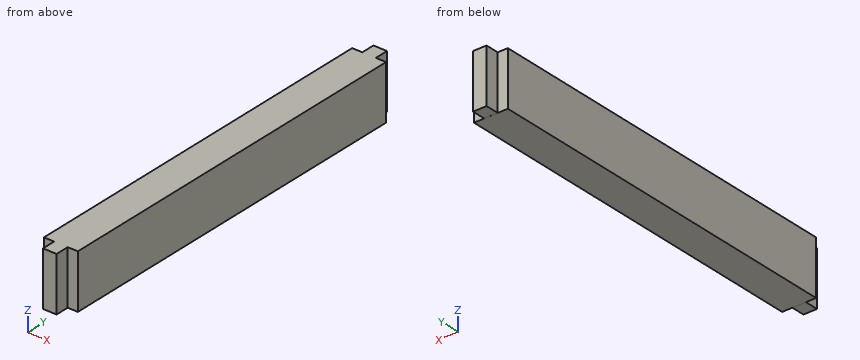
```python
from build123d import *

# Parameters (mm, degrees)
F0_W     = 12.7
F0_H     = 50.77157
F1_DEPTH = 12.7
F2_DEPTH = 365.125
F3_DEPTH = 352.425


with BuildPart() as f1:
    # F0 (on Front) → F1 (new body)
    with BuildSketch(Plane.XZ):
        with Locations((-9.980159, 8.597515)):
            Rectangle(F0_W, F0_H)
    extrude(amount=F1_DEPTH)

    # F0 (on Front) → F2 (join)
    with BuildSketch(Plane.XZ):
        with Locations((-9.980159, 8.597515)):
            Rectangle(F0_W, F0_H)
    extrude(amount=-F2_DEPTH)

    # F0 (on Front) → F3 (join)
    with BuildSketch(Plane.XZ):
        Polygon((-16.330159, 33.9833), (-25.855159, 33.9833), (-25.855159, -16.8167), (5.894841, -16.8167), (5.894841, 33.9833), (-3.630159, 33.9833), (-3.630159, -16.78827), (-16.330159, -16.78827), align=None)
    extrude(amount=-F3_DEPTH)


solid = f1.part
```
CAD build for the part. Positions are in the model's coordinates, mm. Round coordinates to 2 decimals unless told otherwise and drop trailing zeros. Loops run counter-clockwise (first coordinate to the right, second up) from the corner with the lowest first, then second, coordinate; pieces in that order, holes last. Notation, with made-up numbers: M -19,73.5 L -11,73.5 A26 cw -11,105.5 Z; hole C 20.25,-7 d6. An arc over 180 degrees is marked long. Return JSON: item names as keys, results as strings. Group by question number.
(1) Saw through at B-B, the plane x = 2.5. List the corners of the cut face in (y, z) (3 decimals).
(2) Saw through at A-A, the plane z = 6.5. List the corners of the cut face in (x, y) (3 decimals).
(3) Drop flat-ended pins along their axis: P1, Ø4, axis at y = -3.5, z = 8.5, coming from the +X side; P2, Ø6.5, axis at x = -9, y = 357.5, coming from the -Z side; P3, Ø4, axis at y = -7.5, z = 1.5, coming from the -X side. Give the stop position or say it passes through.
(4) Wall check: probe 1 along Y at (x, z) = (2, 11.5) (3 decimals). Give the ranges that are in metal, low to high. Write a range as [from, to].
Answer list:
{
 "1": {"outline": "M 0,-16.817 L 352.425,-16.817 L 352.425,33.983 L 0,33.983 Z"},
 "2": {"outline": "M -25.855,0 L -16.33,0 L -16.33,-12.7 L -3.63,-12.7 L -3.63,0 L 5.895,0 L 5.895,352.425 L -3.63,352.425 L -3.63,365.125 L -16.33,365.125 L -16.33,352.425 L -25.855,352.425 Z"},
 "3": {"P1": "x = -3.63", "P2": "z = -16.79", "P3": "x = -16.33"},
 "4": {"probe 1": "[0, 352.425]"}
}
